Verification items for the finished model (mm, model axes). A direction names the side the tool comes from. Give positions to 0.01 mm unless a question says otherwise; leave off trailing zeros. Order: outer loops, then holes, each group sorted by start corner. A loop starts at its lowest first (then second) coordinate and runs counter-clockwise, first axis right, second up. Notation, with made-up numbers: M 44,25.5 L 99,25.5 A10 ccw 99,39.5 Z; hole C 33,50 d7. An arc over 180 degrees is marked long. Answer as a JSON object with one key per item and string values.
```python
from build123d import *

# Parameters (mm, degrees)
SKETCH_1_R          = 1.5
SKETCH_1_R_2        = 21.5
SKETCH_1_R_3        = 2
EXTRUDE_1_DEPTH     = 15
SKETCH_3_R          = 2.5
SKETCH_3_R_2        = 1.5
CUT_EXTRUDE_1_DEPTH = 16
CUT_EXTRUDE_2_DEPTH = 10
FILLET_1_R          = 1
SKETCH_5_R          = 1.5
SKETCH_5_R_2        = 2.5
SKETCH_5_R_3        = 2
SKETCH_5_R_4        = 32.035606478
EXTRUDE_2_DEPTH     = 15


with BuildPart() as part:
    # 草图1 → 凸台-拉伸1 (new body)
    with BuildSketch(Plane(origin=(0, 0, 0), x_dir=(1, 0, 0), z_dir=(0, 1, 0))):
        with BuildLine():
            Line((21.685248442, 20), (239.195588474, 20))
            ThreePointArc((239.195588474, 20), (248.856506305, 21.719462207), (257.330882485, 26.666666667))
            ThreePointArc((257.330882485, 26.666666667), (315, 0), (257.330882485, -26.666666667))
            ThreePointArc((257.330882485, -26.666666667), (248.856506305, -21.719462207), (239.195588474, -20))
            Line((239.195588474, -20), (21.685248442, -20))
            ThreePointArc((21.685248442, -20), (16.768356723, -20.61381482), (12.153271105, -22.417582418))
            ThreePointArc((12.153271105, -22.417582418), (-25.5, 0), (12.153271105, 22.417582418))
            ThreePointArc((12.153271105, 22.417582418), (16.768356723, 20.61381482), (21.685248442, 20))
        make_face()
        with Locations((302.388176755, -15.969331282)):
            Circle(SKETCH_1_R, mode=Mode.SUBTRACT)
        with Locations((264.030668718, 22.388176755)):
            Circle(SKETCH_1_R, mode=Mode.SUBTRACT)
        with Locations((302.388176755, 15.969331282)):
            Circle(SKETCH_1_R, mode=Mode.SUBTRACT)
        with Locations((264.030668718, -22.388176755)):
            Circle(SKETCH_1_R, mode=Mode.SUBTRACT)
        with Locations((295.969331282, -22.388176755)):
            Circle(SKETCH_1_R, mode=Mode.SUBTRACT)
        with Locations((257.611823245, 15.969331282)):
            Circle(SKETCH_1_R, mode=Mode.SUBTRACT)
        with Locations((257.611823245, -15.969331282)):
            Circle(SKETCH_1_R, mode=Mode.SUBTRACT)
        with Locations((295.969331282, 22.388176755)):
            Circle(SKETCH_1_R, mode=Mode.SUBTRACT)
        with Locations((280, 0)):
            Circle(SKETCH_1_R_2, mode=Mode.SUBTRACT)
        Circle(SKETCH_1_R_3, mode=Mode.SUBTRACT)
        with BuildLine():
            Line((60, 7.5), (200, 7.5))
            ThreePointArc((200, 7.5), (207.5, 0), (200, -7.5))
            Line((200, -7.5), (60, -7.5))
            ThreePointArc((60, -7.5), (52.5, 0), (60, 7.5))
        make_face(mode=Mode.SUBTRACT)
    extrude(amount=EXTRUDE_1_DEPTH)

    # 草图3 → 切除-拉伸1 (cut, through all)
    with BuildSketch(Plane(origin=(0, 15, 0), x_dir=(1, 0, 0), z_dir=(0, 1, 0))):
        with Locations((-5.773502692, -10)):
            Circle(SKETCH_3_R)
        with Locations((-11.547005384, 0)):
            Circle(SKETCH_3_R)
        with Locations((-5.773502692, 10)):
            Circle(SKETCH_3_R)
        with Locations((5.773502692, 10)):
            Circle(SKETCH_3_R)
        with Locations((11.547005384, 0)):
            Circle(SKETCH_3_R)
        with Locations((5.773502692, -10)):
            Circle(SKETCH_3_R)
        with Locations((0, -22.375)):
            Circle(SKETCH_3_R_2)
        with Locations((-19.37731841, -11.1875)):
            Circle(SKETCH_3_R_2)
        with Locations((-19.37731841, 11.1875)):
            Circle(SKETCH_3_R_2)
        with Locations((0, 22.375)):
            Circle(SKETCH_3_R_2)
        with Locations((19.37731841, 11.1875)):
            Circle(SKETCH_3_R_2)
        with Locations((19.37731841, -11.1875)):
            Circle(SKETCH_3_R_2)
    extrude(amount=-CUT_EXTRUDE_1_DEPTH, mode=Mode.SUBTRACT)

    # 草图4 → 切除-拉伸2 (cut)
    with BuildSketch(Plane(origin=(0, 15, 0), x_dir=(1, 0, 0), z_dir=(0, 1, 0))):
        with BuildLine():
            ThreePointArc((283.609642241, 25.697723302), (289.509391905, 25.321470086), (295.398230667, 25.841268715))
            ThreePointArc((295.398230667, 25.841268715), (295.682819381, 25.876430033), (295.969331282, 25.888176755))
            ThreePointArc((295.969331282, 25.888176755), (297.036356329, 25.721562054), (298.001791627, 25.237581069))
            ThreePointArc((298.001791627, 25.237581069), (301.920310217, 21.920310217), (305.237581069, 18.001791627))
            ThreePointArc((305.237581069, 18.001791627), (305.797721775, 16.759902442), (305.841268715, 15.398230667))
            ThreePointArc((305.841268715, 15.398230667), (305.321470086, 9.509391905), (305.697723302, 3.609642241))
            ThreePointArc((305.697723302, 3.609642241), (305.95, 0), (305.697723302, -3.609642241))
            ThreePointArc((305.697723302, -3.609642241), (305.321470086, -9.509391905), (305.841268715, -15.398230667))
            ThreePointArc((305.841268715, -15.398230667), (305.797721775, -16.759902442), (305.237581069, -18.001791627))
            ThreePointArc((305.237581069, -18.001791627), (301.920310217, -21.920310217), (298.001791627, -25.237581069))
            ThreePointArc((298.001791627, -25.237581069), (296.759902442, -25.797721775), (295.398230667, -25.841268715))
            ThreePointArc((295.398230667, -25.841268715), (292.227099274, -25.449471177), (289.034538094, -25.318579131))
            ThreePointArc((289.034538094, -25.318579131), (286.315473672, -25.413480639), (283.609642241, -25.697723302))
            ThreePointArc((283.609642241, -25.697723302), (280, -25.95), (276.390357759, -25.697723302))
            ThreePointArc((276.390357759, -25.697723302), (273.684526328, -25.413480639), (270.965461906, -25.318579131))
            ThreePointArc((270.965461906, -25.318579131), (267.772900726, -25.449471177), (264.601769333, -25.841268715))
            ThreePointArc((264.601769333, -25.841268715), (263.240097558, -25.797721775), (261.998208373, -25.237581069))
            ThreePointArc((261.998208373, -25.237581069), (258.079689783, -21.920310217), (254.762418931, -18.001791627))
            ThreePointArc((254.762418931, -18.001791627), (254.202278225, -16.759902442), (254.158731285, -15.398230667))
            ThreePointArc((254.158731285, -15.398230667), (254.678529914, -9.509391905), (254.302276698, -3.609642241))
            ThreePointArc((254.302276698, -3.609642241), (254.05, 0), (254.302276698, 3.609642241))
            ThreePointArc((254.302276698, 3.609642241), (254.678529914, 9.509391905), (254.158731285, 15.398230667))
            ThreePointArc((254.158731285, 15.398230667), (254.202278225, 16.759902442), (254.762418931, 18.001791627))
            ThreePointArc((254.762418931, 18.001791627), (258.079689783, 21.920310217), (261.998208373, 25.237581069))
            ThreePointArc((261.998208373, 25.237581069), (262.963643671, 25.721562054), (264.030668718, 25.888176755))
            ThreePointArc((264.030668718, 25.888176755), (264.317180619, 25.876430033), (264.601769333, 25.841268715))
            ThreePointArc((264.601769333, 25.841268715), (270.490608095, 25.321470086), (276.390357759, 25.697723302))
            ThreePointArc((276.390357759, 25.697723302), (278.190776366, 25.886853997), (280, 25.95))
            ThreePointArc((280, 25.95), (281.809223634, 25.886853997), (283.609642241, 25.697723302))
        make_face()
    extrude(amount=-CUT_EXTRUDE_2_DEPTH, mode=Mode.SUBTRACT)

    # 圆角1
    fillet_1_edges = [part.edges().sort_by_distance(p)[0] for p in [
        (289.509391905, 5, -25.321470086),
        (296.759902442, 5, -25.797721775),
        (301.920310217, 5, -21.920310217),
        (305.797721775, 5, -16.759902442),
        (305.321470086, 5, -9.509391905),
        (305.95, 5, 0),
        (305.321470086, 5, 9.509391905),
        (305.797721775, 5, 16.759902442),
        (301.920310217, 5, 21.920310217),
        (296.759902442, 5, 25.797721775),
        (289.509391905, 5, 25.321470086),
        (280, 5, 25.95),
        (270.490608095, 5, 25.321470086),
        (263.240097558, 5, 25.797721775),
        (258.079689783, 5, 21.920310217),
        (254.202278225, 5, 16.759902442),
        (254.678529914, 5, 9.509391905),
        (254.05, 5, 0),
        (254.678529914, 5, -9.509391905),
        (254.202278225, 5, -16.759902442),
        (258.079689783, 5, -21.920310217),
        (263.240097558, 5, -25.797721775),
        (270.490608095, 5, -25.321470086),
        (280, 5, -25.95),
    ]]
    fillet(fillet_1_edges, radius=FILLET_1_R)

    # 草图5 → 凸台-拉伸2 (add)
    with BuildSketch(Plane(origin=(0, 15, 0), x_dir=(1, 0, 0), z_dir=(0, 1, 0))):
        with BuildLine():
            Line((-0.75510627, -25.488817441), (15.019724187, -25.956146826))
            ThreePointArc((15.019724187, -25.956146826), (16.500162367, -25.989036105), (17.980925246, -26))
            Line((17.980925246, -26), (241.854825088, -26))
            ThreePointArc((241.854825088, -26), (253.379621277, -27.346335464), (264.283767793, -31.312837088))
            ThreePointArc((264.283767793, -31.312837088), (315.035606478, 0), (264.283767793, 31.312837088))
            ThreePointArc((264.283767793, 31.312837088), (253.379621277, 27.346335464), (241.854825088, 26))
            Line((241.854825088, 26), (17.980925246, 26))
            ThreePointArc((17.980925246, 26), (16.500162367, 25.989036105), (15.019724187, 25.956146826))
            Line((15.019724187, 25.956146826), (-0.75510627, 25.488817441))
            ThreePointArc((-0.75510627, 25.488817441), (-25.5, 0), (-0.75510627, -25.488817441))
        make_face()
        with Locations((0, -22.375)):
            Circle(SKETCH_5_R, mode=Mode.SUBTRACT)
        with Locations((-19.37731841, -11.1875)):
            Circle(SKETCH_5_R, mode=Mode.SUBTRACT)
        with Locations((-5.773502692, -10)):
            Circle(SKETCH_5_R_2, mode=Mode.SUBTRACT)
        with Locations((19.37731841, -11.1875)):
            Circle(SKETCH_5_R, mode=Mode.SUBTRACT)
        with Locations((5.773502692, -10)):
            Circle(SKETCH_5_R_2, mode=Mode.SUBTRACT)
        with Locations((11.547005384, 0)):
            Circle(SKETCH_5_R_2, mode=Mode.SUBTRACT)
        Circle(SKETCH_5_R_3, mode=Mode.SUBTRACT)
        with Locations((-11.547005384, 0)):
            Circle(SKETCH_5_R_2, mode=Mode.SUBTRACT)
        with Locations((-19.37731841, 11.1875)):
            Circle(SKETCH_5_R, mode=Mode.SUBTRACT)
        with Locations((-5.773502692, 10)):
            Circle(SKETCH_5_R_2, mode=Mode.SUBTRACT)
        with Locations((5.773502692, 10)):
            Circle(SKETCH_5_R_2, mode=Mode.SUBTRACT)
        with Locations((19.37731841, 11.1875)):
            Circle(SKETCH_5_R, mode=Mode.SUBTRACT)
        with Locations((0, 22.375)):
            Circle(SKETCH_5_R, mode=Mode.SUBTRACT)
        with Locations((280, 0)):
            Circle(SKETCH_5_R_4, mode=Mode.SUBTRACT)
        with BuildLine():
            Line((60, -7.5), (200, -7.5))
            ThreePointArc((200, -7.5), (207.5, 0), (200, 7.5))
            Line((200, 7.5), (60, 7.5))
            ThreePointArc((60, 7.5), (52.5, 0), (60, -7.5))
        make_face(mode=Mode.SUBTRACT)
    extrude(amount=-EXTRUDE_2_DEPTH)


solid = part.part
```
Q1. Release check for a two-part mould opening along X. For faces 1 (the face through (253.22, 7.6, 27.31)), 2 (the face through (128, 8, 26)), 3 (the face through (254.05, 10.56, 0.05)), 4 (the face through (207.5, 7.4, -0.16)) record: +X half, -X half, draft (parallel to the pull), parting line (faces both ways), or undercut.
Resolved:
{"face 1": "-X half", "face 2": "draft", "face 3": "undercut", "face 4": "undercut"}
Q2. Section check C-C on y = 11.25. Count the separate pieces of the cut face and the enclosed holes in it, then the cut area to 3 significant figures.
Resolved:
{"separate pieces": "1", "enclosed holes": "15", "area": "12,900 mm²"}
Q3. Gauge pin test, flat ends, axial feed: pin 1 Ø8 at (x, z) = (-5.77, 10) entering from -Y; pin 2 Ø4 at (x, z) = (295.97, -22.39) entering from +Y; pin 3 Ø4 at (y, z) = (5.5, 21) entering from +X; pin 4 Ø4 at (y, z) = (7.5, 5.5) entering from +X. Record the tip position at first contact, or that the pin passes through.
Resolved:
{"pin 1": "stops at y = 0", "pin 2": "stops at y = 5", "pin 3": "stops at x = 309.44", "pin 4": "stops at x = 314.86"}
Q4. Section check B-B on x = 46.5. Record the cut outline in (y, z).
Resolved:
{"outline": "M 0,-26 L 15,-26 L 15,26 L 0,26 Z"}
Q5. Section check A-A on x = 110. Record the cut outline in (y, z), then the cut area to 3 significant figures.
Resolved:
{"outline": "M 0,-26 L 15,-26 L 15,-7.5 L 0,-7.5 Z; M 0,7.5 L 15,7.5 L 15,26 L 0,26 Z", "area": "555 mm²"}
Q6. Tool access check on faces 5 (the face through (287.5, 5, -20.4)), 6 (the face through (131, 7, 7.5)). Record the directions out of +Z, -Z, +X, -X, +Y, -Y that give a thin tool (end or side, any length) a straight path to the whole face; none if there is none.
Resolved:
{"face 5": "+Y", "face 6": "+Y, -Y"}
Q7. Material ranges on L1, parallel to Z at x = 4, y = 1.75; L2, parallel to X at y = 13.5, z = -1; L3, parallel to Z at x = 189.5, y = 10.5, recorded low to high.
Resolved:
{"L1": "z = -25.63 to -11.76, -8.24 to 8.24, 11.76 to 25.63", "L2": "x = -25.48 to -13.84, -9.26 to -1.73, 1.73 to 9.26, 13.84 to 52.57, 207.43 to 254.07, 305.93 to 315.02", "L3": "z = -26 to -7.5, 7.5 to 26"}
